Can you work these out from the model? Positions are in its coordinate system, mm. A direction names the side the tool comes from. Give positions to 0.01 mm unless a question says otherwise; leave off trailing zeros. Loops run counter-clockwise (first coordinate to the right, second up) from the corner with the lowest first, then second, coordinate; pieces in that order, holes last. Notation, with made-up numbers: (-25.75, 38) - (29.25, 38) arc R19 ccw to (29.25, 49) - close; hole circle Ø8 at (-26.5, 78). An arc over 180 degrees is marked (long way). Answer in a Markdown table with one row per item.
from build123d import *

# Parameters (mm, degrees)
BOSS_EXTRU_2_DEPTH         = 10
CONG_1_R                   = 10
D_GAGEMENT_M81_D           = 9
D_GAGEMENT_M81_CSINK_D     = 9.05
D_GAGEMENT_M81_CSINK_ANGLE = 90
D_GAGEMENT_M61_D           = 6.6


with BuildPart() as part:
    # Esquisse1 → Boss.-Extru.2 (new body)
    with BuildSketch(Plane.XY):
        with BuildLine():
            Line((-7, 38), (-7, -38))
            ThreePointArc((-7, -38), (0, -57.485281374), (7, -38))
            Line((7, -38), (7, 38))
            ThreePointArc((7, 38), (0, 57.485281374), (-7, 38))
        make_face()
    extrude(amount=BOSS_EXTRU_2_DEPTH)

    # Congé1
    cong_1_edges = [part.edges().sort_by_distance(p)[0] for p in [
        (7, 38, 5),
        (7, -38, 5),
        (-7, -38, 5),
        (-7, 38, 5),
    ]]
    fillet(cong_1_edges, radius=CONG_1_R)

    # Dégagement M81 (through all)
    with Locations(Plane.XY.offset(10)):
        with Locations((0, -46.485281374)):
            CounterSinkHole(D_GAGEMENT_M81_D / 2, D_GAGEMENT_M81_CSINK_D / 2, counter_sink_angle=D_GAGEMENT_M81_CSINK_ANGLE)

    # Dégagement M61 (through all)
    with Locations(Plane.XY.offset(10)):
        with Locations((0, 46.485281374)):
            Hole(D_GAGEMENT_M61_D / 2)


solid = part.part
Q1. If we mould it in two halves opening along X, with no side actions, what happens to faces 1 (the face through (0, 1, 10)), 2 (the face through (7.5, -37.28, 5.07)), 3 (the face through (-1.77, 49.27, 4.93)), 4 (the face through (0.976, -50.878, 4.918))? For each: released by +X, released by -X, zero draft, split by the parting line, or undercut.
Checked values:
| item | result |
|---|---|
| face 1 | zero draft |
| face 2 | released by +X |
| face 3 | undercut |
| face 4 | undercut |
Q2. Imagine slicing it at D-D, the plane y = 37. Write out the boundary of the cut face in (x, z), and give its area (3 significant figures).
Checked values:
| item | result |
|---|---|
| outline | (-7.41, 0) - (7.41, 0) - (7.41, 10) - (-7.41, 10) - close |
| area | 148 mm² |
Q3. If I drill on line 1 (Y direction, x = 0, z = 5.25); line 2 (Y direction, x = 1, z = 4.75); line 3 (X direction, y = -2, z = 8.25), over which ranges is the centre line in solid material (lowest first)? Write a range as [from, to].
Checked values:
| item | result |
|---|---|
| line 1 | y = [-57.49, -50.99], [-41.99, 43.19], [49.79, 57.49] |
| line 2 | y = [-57.44, -50.87], [-42.1, 43.34], [49.63, 57.44] |
| line 3 | x = [-7, 7] |
Q4. For pin 1 (1 mm diameter, centred on y = -26, z = 8, fed in from +X); pin 2 (1 mm diameter, centred on y = 29, z = 3, fed in from -X); pin 3 (2 mm diameter, centred on x = 2, z = 6.5, fed in from -Y), each with a flat end and sliding along its axis, tell me the tip position at first contact or that it passes through.
Checked values:
| item | result |
|---|---|
| pin 1 | stops at x = 7 |
| pin 2 | stops at x = -7 |
| pin 3 | stops at y = -57.44 |
Q5. On a 3-axis mill with a long thin cutter (end or side, diameter ignored), from which of +Z, -Z, +X, -X, +Y, -Y can I reach the whole of each face in a straight line? I mean faces 5 (the face through (7.475, 37.201, 5.07)), 6 (the face through (-7, 0, 5)), 7 (the face through (-0.34, -57.48, 4.93)). Say none if no direction works.
Checked values:
| item | result |
|---|---|
| face 5 | +Z, -Z, +X |
| face 6 | +Z, -Z, -X |
| face 7 | +Z, -Z |
Q6. Imagine slicing it at A-A, the plane x = 0. Write out the boundary of the cut face in (y, z) (3 decimals).
Checked values:
| item | result |
|---|---|
| outline | (-57.485, 0) - (-50.985, 0) - (-50.985, 9.975) - (-51.01, 10) - (-57.485, 10) - close; (-41.985, 0) - (43.185, 0) - (43.185, 10) - (-41.96, 10) - (-41.985, 9.975) - close; (49.785, 0) - (57.485, 0) - (57.485, 10) - (49.785, 10) - close |
Q7. Imagine slicing it at C-C, the plane y = -27.5. Write out the boundary of the cut face in (x, z).
Checked values:
| item | result |
|---|---|
| outline | (-7, 0) - (7, 0) - (7, 10) - (-7, 10) - close |
Q8. Imagine slicing it at B-B, the plane z = 7.5. Write out the boundary of the cut face in (x, y), and give its area (3 significant figures).
Checked values:
| item | result |
|---|---|
| outline | (-8.9, -40.03) arc R11 ccw (long way) to (8.9, -40.03) arc R10 cw to (7, -34.16) - (7, 34.16) arc R10 cw to (8.9, 40.03) arc R11 ccw (long way) to (-8.9, 40.03) arc R10 cw to (-7, 34.16) - (-7, -34.16) arc R10 cw to start; hole circle Ø9 at (0, -46.49); hole circle Ø6.6 at (0, 46.49) |
| area | 1,680 mm² |
